Source: CAD feature listing. Evaluate the final solid. Frame: model axes, mm. Face numbers are marked on the shaded views. A direction names the side the tool comes from. Round coordinates to 2 decimals unless told otherwise and drop trailing zeros. Order: outer loops, then holes, each group sorted by start corner. A loop starts at its lowest first (then second) coordinate and runs counter-clockwise, first axis right, second up. Notation, with made-up numbers: (-16.75, 88.5) -> (13.25, 88.5) arc R23 ccw to (13.25, 100.5) -> close; hole circle Ø5 at (37.5, 40.25). An arc over 180 degrees is marked (long way). Answer as CSV lines item,"result". Start each with the question number.
(1) Contact query for flat-ended pins moving along their axis: P1, Ø1.5, axis at x = 5.5, y = 41.5, coming from the +Z side; P2, Ø8, axis at x = -4.5, y = 39, coming from the +Z side; P3, Ø8, axis at x = -0.5, y = 33.5, coming from the -Z side; P4, Ø11, axis at x = 1, z = 3, coming from the +Y side. Output: stop coordinate, or through.
(2) Section query C-C (y = 42.5). Output: boundary loops of the cut face in (x, z).
(3) Set-up query: the marked faces 1 and 2. Return all of +Z, -Z, +X, -X, +Y, -Y with unobstructed straight access to the full face (end or side cutting, diameter ignored); none if empty.
(4) Section query B-B (x = -8.5). Count the separate pieces of the cut face and the enclosed holes in it, plus the area to 3 significant figures.
(5) Section query A-A (y = 4.5). Output: boundary loops of the cut face in (x, z), plus the area to 3 significant figures.
(6) Pull-direction query (X, two-part tool) for the marked faces 3, 4 and 5; classes: +X half, -X half, draft (parallel to the pull), parting line (faces both ways), or undercut.
(7) Line query: line 1 along X through (y, z) = (32.95, 0); line 2 along X through (y, z) = (11.5, -2); line 3 along Z through (x, y) = (-4, 19.5). Output: solid intervals per line, ascending. Write a range as from..to.
```python
from build123d import *


with BuildPart() as part:
    # Sketch1 → Revolve1 (revolve)
    with BuildSketch(Plane.XY, mode=Mode.PRIVATE) as revolve1_sk:
        Polygon((0, 0), (11.15, 0), (11.15, 1), (5.5, 1), (5.5, 2.5), (11.15, 2.5), (11.15, 3.5), (5.4, 3.5), (5.4, 5), (11.15, 5), (11.15, 6), (5.3, 6), (5.3, 7.5), (11.15, 7.5), (11.15, 8.5), (5.2, 8.5), (5.2, 10), (11.15, 10), (11.15, 11), (5.1, 11), (5.1, 12.5), (11.15, 12.5), (11.15, 13.5), (5, 13.5), (5, 15), (11.15, 15), (11.15, 16), (4.9, 16), (4.9, 17.5), (11.15, 17.5), (11.15, 18.5), (4.8, 18.5), (4.8, 20), (11.15, 20), (11.15, 21), (4.7, 21), (4.7, 22.5), (11.15, 22.5), (11.15, 23.5), (4.6, 23.5), (4.6, 25), (11.15, 25), (11.15, 26), (4.5, 26), (4.5, 27.5), (8, 27.5), (8, 28.5), (4.4, 28.5), (4.4, 30), (8, 30), (8, 33), (6, 33), (6, 39), (8, 39), (8, 46), (0, 46), align=None)
    revolve(revolve1_sk.sketch.rotate(Axis((0, 0, 0), (0, 1, 0)), 90), axis=Axis((0, 0, 0), (0, 1, 0)))

    # Sketch2 → Cut-Revolve1 (revolve, cut)
    with BuildSketch(Plane.XY, mode=Mode.PRIVATE) as cut_revolve1_sk:
        Polygon((0, 46), (6.75, 46), (6.75, 40.5), (5, 39.489637029), (5, 36.489637029), (3.25, 35.479274058), (3.25, 31.5), (1.6, 30.547372056), (1.6, 18.519615242), (2.5, 18), (2.5, 14), (3, 14), (3, 0), (0, 0), align=None)
    revolve(cut_revolve1_sk.sketch.rotate(Axis((0, 0, 0), (0, 1, 0)), 90), axis=Axis((0, 0, 0), (0, 1, 0)), mode=Mode.SUBTRACT)


solid = part.part
```
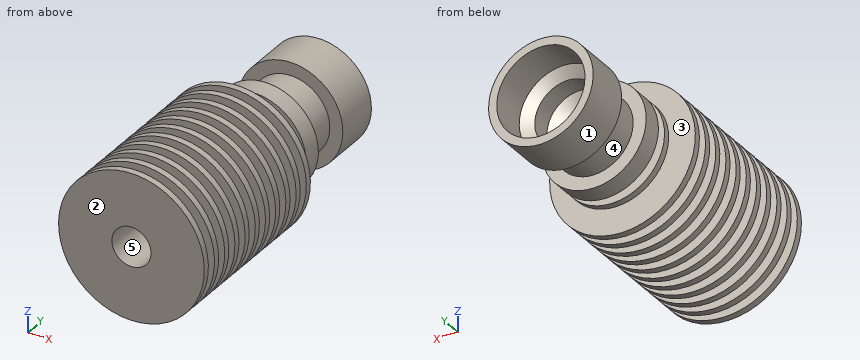
Answer block:
1,P1,"z = 6.44"
1,P2,"z = 7.98"
1,P3,"z = -8"
1,P4,"y = 46"
2,outline,"circle Ø16 at (0, 0); hole circle Ø13.5 at (0, 0)"
3,face 1,"+Y"
3,face 2,"+Z, -Z, +X, -X, -Y"
4,separate pieces,"11"
4,enclosed holes,"0"
4,area,"159 mm2"
5,outline,"circle Ø10.8 at (0, 0); hole circle Ø6 at (0, 0)"
5,area,"63.3 mm2"
6,face 3,"draft"
6,face 4,"parting line"
6,face 5,"undercut"
7,line 1,"-8..-3.25, 3.25..8"
7,line 2,"-4.69..-2.24, 2.24..4.69"
7,line 3,"-2.65..2.65"
